```python
from build123d import *

# Parameters (mm, degrees)
SKETCH1_W                                           = 55
SKETCH1_H                                           = 88
BOSS_EXTRUDE1_DEPTH                                 = 10
M5_TAPPED_HOLE1_D                                   = 4.2
CBORE_FOR_M5_HEX_SOCKET_HEAD_CAP_SCREW1_D           = 5.5
CBORE_FOR_M5_HEX_SOCKET_HEAD_CAP_SCREW1_CBORE_D     = 10
CBORE_FOR_M5_HEX_SOCKET_HEAD_CAP_SCREW1_CBORE_DEPTH = 5.4


with BuildPart() as part:
    # Sketch1 → Boss-Extrude1 (new body)
    with BuildSketch(Plane.XY):
        Rectangle(SKETCH1_W, SKETCH1_H)
    extrude(amount=BOSS_EXTRUDE1_DEPTH)

    # M5 Tapped Hole1 (through all)
    with Locations(Plane.XY.offset(10)):
        with Locations((-17.5, 17), (6.5, 17), (-17.5, -17), (6.5, -17)):
            Hole(M5_TAPPED_HOLE1_D / 2)

    # CBORE for M5 Hex Socket Head Cap Screw1 (through all)
    with Locations(Plane.XY.offset(10)):
        with Locations((5.5, 30), (17.5, 30), (17.5, -30), (5.5, -30)):
            CounterBoreHole(CBORE_FOR_M5_HEX_SOCKET_HEAD_CAP_SCREW1_D / 2, CBORE_FOR_M5_HEX_SOCKET_HEAD_CAP_SCREW1_CBORE_D / 2, CBORE_FOR_M5_HEX_SOCKET_HEAD_CAP_SCREW1_CBORE_DEPTH)


solid = part.part
```
Part model, mm, in its own coordinate system. A direction names the side the tool comes from. Round coordinates to 2 decimals unless told otherwise and drop trailing zeros. Write each loop counter-clockwise with the first axis right and the second up, starting at its lowest first coordinate (ties: lowest second). Pieces come first, ordered by that corner, then holes. Notation, with made-up numbers: M 41.5,13.5 L 95.5,13.5 A35 cw 95.5,46.5 Z; hole C 7.5,40.5 d8. An arc over 180 degrees is marked long. One line per question, with ' | ' between items.
(1) Saw through at B-B on x = 17.5. Write the cut outline in (y, z), then the cut area to 3 significant figures.
Answer key:
outline: M -44,0 L -32.75,0 L -32.75,4.6 L -35,4.6 L -35,10 L -44,10 Z; M -27.25,0 L 27.25,0 L 27.25,4.6 L 25,4.6 L 25,10 L -25,10 L -25,4.6 L -27.25,4.6 Z; M 32.75,0 L 44,0 L 44,10 L 35,10 L 35,4.6 L 32.75,4.6 Z | area: 721 mm^2
(2) Saw through at D-D on x = 6.5. Write the cut outline in (y, z).
Answer key:
outline: M -44,0 L -32.56,0 L -32.56,4.6 L -34.9,4.6 L -34.9,10 L -44,10 Z; M -27.44,0 L -19.1,0 L -19.1,10 L -25.1,10 L -25.1,4.6 L -27.44,4.6 Z; M -14.9,0 L 14.9,0 L 14.9,10 L -14.9,10 Z; M 19.1,0 L 27.44,0 L 27.44,4.6 L 25.1,4.6 L 25.1,10 L 19.1,10 Z; M 32.56,0 L 44,0 L 44,10 L 34.9,10 L 34.9,4.6 L 32.56,4.6 Z
(3) 3-axis set-ups, long thin cutter, end or side, ignore diameter. For faces 4 (the face through (8, -32, 4.6)), 5 (the face through (27.5, -1, 5)): which of +Z, -Z, +X, -X, +Y, -Y reach the whole face in a straight line?
Answer key:
face 4: +Z | face 5: +Z, -Z, +X, +Y, -Y
(4) Two-plate mould, pull along X, no slides. Class faces 1 (the face through (4.42, -34.88, 7.34)), 2 (the face through (0, 1, 0)), 3 (the face through (-27.5, -1, 5)): released by +X, released by -X, zero draft, split by the parting line, or undercut.
Answer key:
face 1: undercut | face 2: zero draft | face 3: released by -X
(5) Saw through at C-C on z = 3. Count the separate pieces of the cut face and the enclosed holes in it, then the cut area to 3 significant figures.
Answer key:
separate pieces: 1 | enclosed holes: 8 | area: 4,690 mm^2
(6) Saw through at A-A on y = 17. Write the cut outline in (x, z), then the cut area to 3 significant figures.
Answer key:
outline: M -27.5,0 L -19.6,0 L -19.6,10 L -27.5,10 Z; M -15.4,0 L 4.4,0 L 4.4,10 L -15.4,10 Z; M 8.6,0 L 27.5,0 L 27.5,10 L 8.6,10 Z | area: 466 mm^2
(7) Probe line 1 along Y through (x, z) = (17.5, 6.05); line 2 along Y through (x, z) = (-17.5, 4); line 3 along X through (y, z) = (-29, 7). List the from-to ranges inside material, lowest first.
Answer key:
line 1: y = -44 to -35, -25 to 25, 35 to 44 | line 2: y = -44 to -19.1, -14.9 to 14.9, 19.1 to 44 | line 3: x = -27.5 to 0.6, 10.4 to 12.6, 22.4 to 27.5
